Could you check a few things on this model? Use its own coordinates, in mm. Face numbers are marked on the shaded views. A direction names the side the tool comes from. Round coordinates to 2 decimals unless told otherwise and drop trailing zeros. Loops run counter-clockwise (first coordinate to the right, second up) from the corner with the lowest first, then second, coordinate; pieces in that order, holes last. Notation, with made-up numbers: M 32.5,-35 L 59.5,-35 A20 cw 59.5,0 Z; hole C 55.5,29.25 d11. An arc over 180 degrees is marked long. One line per item, written item: value. Start each with the question number.
Q1. Which directions (+Z, -Z, +X, -X, +Y, -Y) give clear straight access to the entire face, cutting with the end or side of a thin tool? Please do the marked faces 4 and 5.
Q2. Please list where these lines run through material, in increasing order: line 1 along Z through (x, y) = (0, 29); line 2 along Y through (x, z) = (-2, 3); line 3 along X through (y, z) = (18, 4.25).
Q3. Imagine slicing it at A-A (y = -12). Please give me the cut outline in (x, z).
Q4. Imagine slicing it at C-C (z = 10). Give the number of separate pieces and of enclosed holes in the cut face, then the cut area to 3 significant figures.
Q5. Imagine slicing it at B-B (x = 25). Please give me the cut outline in (y, z), then the cut area to 3 significant figures.
Q6. Imagine slicing it at D-D (z = 4.75). Please give me the cut outline in (x, y).
Q7. Thinking about a two-plate mould opening in Y: for the marked faces 1, 2 and 3, which applies, released by +Y, released by -Y, zero draft, split by the parting line, or undercut?
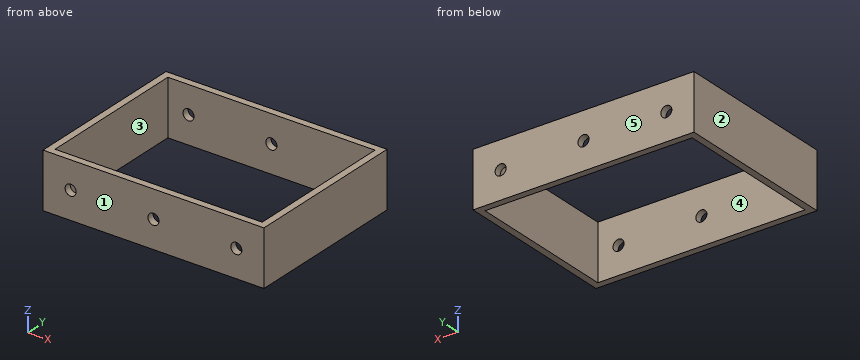
from build123d import *

# Parameters (mm, degrees)
F0_W     = 80
F0_H     = 60
F1_DEPTH = 20
F2_W     = 75
F2_H     = 55
F3_DEPTH = 20.001
F4_R     = 2
F5_DEPTH = 60.001


with BuildPart() as f1:
    # F0 (on Top) → F1 (new body)
    with BuildSketch(Plane.XY):
        Rectangle(F0_W, F0_H)
    extrude(amount=F1_DEPTH)

    # F2 (on face) → F3 (cut, through all)
    with BuildSketch(Plane.XY.offset(20)):
        Rectangle(F2_W, F2_H)
    extrude(amount=-F3_DEPTH, mode=Mode.SUBTRACT)

    # F4 (on face) → F5 (cut, through all)
    with BuildSketch(Plane.XZ.offset(30)):
        with Locations((-30, 10)):
            Circle(F4_R)
        with Locations((0, 10)):
            Circle(F4_R)
        with Locations((30, 10)):
            Circle(F4_R)
    extrude(amount=-F5_DEPTH, mode=Mode.SUBTRACT)


solid = f1.part
Report:
1. face 4: +Z, -Z
1. face 5: +Z, -Z, +X, -X, +Y
2. line 1: z = 0 to 8, 12 to 20
2. line 2: y = -30 to -27.5, 27.5 to 30
2. line 3: x = -40 to -37.5, 37.5 to 40
3. outline: M -40,0 L -37.5,0 L -37.5,20 L -40,20 Z; M 37.5,0 L 40,0 L 40,20 L 37.5,20 Z
4. separate pieces: 6
4. enclosed holes: 0
4. area: 615 mm²
5. outline: M -30,0 L -27.5,0 L -27.5,20 L -30,20 Z; M 27.5,0 L 30,0 L 30,20 L 27.5,20 Z
5. area: 100 mm²
6. outline: M -40,-30 L 40,-30 L 40,30 L -40,30 Z; hole M -37.5,-27.5 L 37.5,-27.5 L 37.5,27.5 L -37.5,27.5 Z
7. face 1: released by -Y
7. face 2: zero draft
7. face 3: undercut
